Can you work these out from the model? Positions are in its coordinate system, mm. A direction names the side the tool comes from. Coordinates: 2 decimals unless noted, no trailing zeros. Order: outer loops, then holes, each group sorted by start corner. A loop starts at its lowest first (then second) coordinate and runs counter-clockwise, first axis right, second up. Notation, with made-up numbers: (9.5, 14) -> (37.5, 14) arc R20 ccw to (37.5, 45) -> close; hole circle Ø4 at (-37.5, 53.5). An arc over 180 degrees is marked (long way). Return JSON: item names as keys, results as strings. Group by question number.
1) For faces 5 (the cylindrical face through (-0.2, 161.4, 12.7)), 6 (the cylindrical face through (-0.18, 161.35, -11.11)), which set-ups out of +Z, -Z, +X, -X, +Y, -Y let a thin tool reach every point of the face, with its end or its side?
2) For pin 1 (8 mm diameter, centred on x = 9, z = -3.5, fed in from +Y); pin 2 (8 mm diameter, centred on x = -2, z = -4.5, fed in from +Y), each with a flat end and sliding along its axis, tell me the tip position at first contact or that it passes through.
3) If we section it at A-A, the plane z = 0: Please give me the cut outline in (x, y) (3 decimals).
4) If we section it at C-C, the plane x = -2.75: Please give me the cut outline in (y, z).
5) Thinking about a two-plate mould opening in Y: for faces 1 (the flat face through (10.087, 161, 0)), 2 (the flat face through (-10.4, 0, 0.9)), 3 (the flat face through (-10.4, 327.29, 0.9)), 4 (the cylindrical face through (-10.87, 310.69, 0.41)), which applies, +Y half, -Y half, draft (parallel to the pull), parting line (faces both ways), or undercut?
6) If I drill on probe 1 along Y at (x, z) = (-10.7, 0) (3 decimals); probe 2 along Z at (x, y) = (-0.5, 14); probe 3 along X at (y, z) = (167, 4.25), over which ranges is the centre line in solid material (lowest first)? Write a range as from..to.
7) If we section it at D-D, the plane y = 174: Please give me the cut outline in (x, z) (1 decimal), then the cut area to 3 significant figures.
8) If we section it at B-B, the plane y = 21.5: Please give me the cut outline in (x, z) (1 decimal), then the cut area to 3 significant figures.
from build123d import *

# Parameters (mm, degrees)
BOSS_EXTRUDE1_DEPTH = 327.29
CUT_EXTRUDE1_REACH  = 330.367
SKETCH2_R           = 3.175


with BuildPart() as part:
    # Sketch1 → Boss-Extrude1 (new body)
    with BuildSketch(Plane(origin=(0, 0, 0), x_dir=(1, 0, 0), z_dir=(0, 1, 0))):
        with BuildLine():
            Line((11.674330816, -5), (11.674330816, 5))
            ThreePointArc((11.674330816, 5), (0, 12.7), (-11.674330816, 5))
            Line((-11.674330816, 5), (-11.674330816, -5))
            ThreePointArc((-11.674330816, -5), (0, -12.7), (11.674330816, -5))
        make_face()
        with BuildLine():
            Line((10.086830816, 4.662992638), (10.086830816, -4.662992638))
            ThreePointArc((10.086830816, -4.662992638), (0, -11.1125), (-10.086830816, -4.662992638))
            Line((-10.086830816, -4.662992638), (-10.086830816, 4.662992638))
            ThreePointArc((-10.086830816, 4.662992638), (0, 11.1125), (10.086830816, 4.662992638))
        make_face(mode=Mode.SUBTRACT)
    extrude(amount=BOSS_EXTRUDE1_DEPTH)

    # Cut-Extrude1: up to this face of the body (flat: up to its plane)
    cut_extrude1_end = Plane(part.part.faces().sort_by_distance((-11.674330816, 163.645, 0))[0])
    # Sketch2 → Cut-Extrude1 (cut, up to the picked face)
    with BuildSketch(Plane(origin=(11.674330816, 0, 0), x_dir=(0, 0, -1), z_dir=(1, 0, 0)), mode=Mode.PRIVATE) as cut_extrude1_sk1:
        with Locations((0, 21.5)):
            Circle(SKETCH2_R)
    cut_extrude1_tool1 = split(extrude(cut_extrude1_sk1.sketch, amount=-CUT_EXTRUDE1_REACH, mode=Mode.PRIVATE), bisect_by=cut_extrude1_end, keep=Keep.BOTH, mode=Mode.PRIVATE)
    # Sketch2 → Cut-Extrude1 (cut, up to the picked face)
    with BuildSketch(Plane(origin=(11.674330816, 0, 0), x_dir=(0, 0, -1), z_dir=(1, 0, 0)), mode=Mode.PRIVATE) as cut_extrude1_sk2:
        with Locations((0, 307.54)):
            Circle(SKETCH2_R)
    cut_extrude1_tool2 = split(extrude(cut_extrude1_sk2.sketch, amount=-CUT_EXTRUDE1_REACH, mode=Mode.PRIVATE), bisect_by=cut_extrude1_end, keep=Keep.BOTH, mode=Mode.PRIVATE)
    add(cut_extrude1_tool1.solids().sort_by(Axis((11.674331, 21.5, 0), (-1, 0, 0)))[0], mode=Mode.SUBTRACT)
    add(cut_extrude1_tool2.solids().sort_by(Axis((11.674331, 307.54, 0), (-1, 0, 0)))[0], mode=Mode.SUBTRACT)


solid = part.part
Result sheet:
{
 "1": {"face 5": "+Z, +Y, -Y", "face 6": "+Y, -Y"},
 "2": {"pin 1": "stops at y = 327.29", "pin 2": "passes through"},
 "3": {"outline": "(-11.674, 0) -> (-10.087, 0) -> (-10.087, 18.325) -> (-11.674, 18.325) -> close; (-11.674, 24.675) -> (-10.087, 24.675) -> (-10.087, 304.365) -> (-11.674, 304.365) -> close; (-11.674, 310.715) -> (-10.087, 310.715) -> (-10.087, 327.29) -> (-11.674, 327.29) -> close; (10.087, 0) -> (11.674, 0) -> (11.674, 18.325) -> (10.087, 18.325) -> close; (10.087, 24.675) -> (11.674, 24.675) -> (11.674, 304.365) -> (10.087, 304.365) -> close; (10.087, 310.715) -> (11.674, 310.715) -> (11.674, 327.29) -> (10.087, 327.29) -> close"},
 "4": {"outline": "(0, -12.4) -> (327.29, -12.4) -> (327.29, -10.77) -> (0, -10.77) -> close; (0, 10.77) -> (327.29, 10.77) -> (327.29, 12.4) -> (0, 12.4) -> close"},
 "5": {"face 1": "draft", "face 2": "-Y half", "face 3": "+Y half", "face 4": "undercut"},
 "6": {"probe 1": "y = 0..18.325, 24.675..304.365, 310.715..327.29", "probe 2": "z = -12.69..-11.1, 11.1..12.69", "probe 3": "x = -11.67..-10.09, 10.09..11.67"},
 "7": {"outline": "(-11.7, -5) arc R12.7 ccw to (11.7, -5) -> (11.7, 5) arc R12.7 ccw to (-11.7, 5) -> close; hole (-10.1, -4.7) arc R11.1 ccw to (10.1, -4.7) -> (10.1, 4.7) arc R11.1 ccw to (-10.1, 4.7) -> close", "area": "118 mm2"},
 "8": {"outline": "(-11.7, -5) arc R12.7 ccw to (11.7, -5) -> (11.7, -3.2) -> (10.1, -3.2) -> (10.1, -4.7) arc R11.1 cw to (-10.1, -4.7) -> (-10.1, -3.2) -> (-11.7, -3.2) -> close; (-11.7, 3.2) -> (-10.1, 3.2) -> (-10.1, 4.7) arc R11.1 cw to (10.1, 4.7) -> (10.1, 3.2) -> (11.7, 3.2) -> (11.7, 5) arc R12.7 ccw to (-11.7, 5) -> close", "area": "97.7 mm2"}
}
